Source: CAD feature listing. Evaluate the final solid. Frame: model axes, mm. A direction names the side the tool comes from. Round coordinates to 2 decimals unless told otherwise and drop trailing zeros. Order: outer loops, then holes, each group sorted by start corner. A loop starts at its lowest first (then second) coordinate and runs counter-clockwise, first axis right, second up. Notation, with made-up numbers: (-30, 19) -> (-4, 19) arc R20 cw to (-4, 39) -> close; hole circle Ø10 at (30.5, -7.75). An arc over 180 degrees is marked (long way). Answer as CSV lines item,"result".
from build123d import *

# Parameters (mm, degrees)
SKETCH1_W           = 17
SKETCH1_H           = 15
BOSS_EXTRUDE1_DEPTH = 81
CUT_EXTRUDE1_DEPTH  = 40
SKETCH3_R           = 1.5
CUT_EXTRUDE2_DEPTH  = 36
SKETCH4_W           = 17
SKETCH4_H           = 7
BOSS_EXTRUDE2_DEPTH = 14
SKETCH5_R           = 2
CUT_EXTRUDE3_DEPTH  = 14


with BuildPart() as part:
    # Sketch1 → Boss-Extrude1 (new body)
    with BuildSketch(Plane(origin=(0, 0, 0), x_dir=(1, 0, 0), z_dir=(0, 1, 0))):
        with Locations((-68.404761905, 8.571428571)):
            Rectangle(SKETCH1_W, SKETCH1_H)
    extrude(amount=BOSS_EXTRUDE1_DEPTH)

    # Sketch2 → Cut-Extrude1 (cut)
    with BuildSketch(Plane(origin=(-59.904761905, 0, 0), x_dir=(0, 0, -1), z_dir=(1, 0, 0))):
        Polygon((16.071428571, 0), (1.071428571, 0), (1.071428571, 6.994614872), align=None)
    extrude(amount=-CUT_EXTRUDE1_DEPTH, mode=Mode.SUBTRACT)

    # Sketch3 → Cut-Extrude2 (cut)
    with BuildSketch(Plane(origin=(0, 6.155714275, -2.870456708), x_dir=(1, 0, 0), z_dir=(0, -0.9063077870366528, 0.4226182617406934))):
        with Locations(Location((-68.404761905, -5.514992079, 0), (0, 0, 270))):
            Circle(SKETCH3_R)
    extrude(amount=-CUT_EXTRUDE2_DEPTH, mode=Mode.SUBTRACT)

    # Sketch4 → Boss-Extrude2 (add)
    with BuildSketch(Plane(origin=(0, 0, -16.071428571), x_dir=(-1, 0, 0), z_dir=(0, 0, -1))):
        with Locations((68.404761905, 77.5)):
            Rectangle(SKETCH4_W, SKETCH4_H)
    extrude(amount=BOSS_EXTRUDE2_DEPTH)

    # Sketch5 → Cut-Extrude3 (cut)
    with BuildSketch(Plane(origin=(0, 74, 0), x_dir=(-1, 0, 0), z_dir=(0, -1, 0))):
        with Locations(Location((71.904761905, 23.071428571, 0), (0, 0, 90))):
            Circle(SKETCH5_R)
        with Locations(Location((64.904761905, 23.071428571, 0), (0, 0, 90))):
            Circle(SKETCH5_R)
    extrude(amount=-CUT_EXTRUDE3_DEPTH, mode=Mode.SUBTRACT)


solid = part.part
1. Mould query, pull axis X, two halves, no side actions, for faces 1 (the flat face through (-59.905, 49, -9)), 2 (the flat face through (-76.905, 49, -9)), 3 (the cylindrical face through (-68.339, 12.335, -10.184)), 4 (the cylindrical face through (-66.857, 77.451, -22.638)). Classes: released by +X, released by -X, zero draft, split by the parting line, or undercut.
Results below:
face 1,"released by +X"
face 2,"released by -X"
face 3,"undercut"
face 4,"undercut"
2. Section query C-C on y = 59. Return loops of the section in (x, z).
Results below:
outline,"(-76.9, -16.07) -> (-59.9, -16.07) -> (-59.9, -1.07) -> (-76.9, -1.07) -> close"
3. Reachability of faces 5 (the cylindrical face through (-73.857, 77.451, -22.638)), 6 (the flat face through (-68, 74, -23)) from +Z, -Z, +X, -X, +Y, -Y: full face, straight path, thin tool, end or side. Return the list, or none.
Results below:
face 5,"+Y, -Y"
face 6,"-Z, +X, -X, -Y"
4. Line query: L1, parallel to Y at x = -68, z = -22.75; L2, parallel to Z at x = -63.5, y = 31.5; L3, parallel to Z at x = -67.25, y = 4.5. Output: solid intervals per line, ascending. Write a range as [from, to].
Results below:
L1,"[74, 81]"
L2,"[-16.07, -1.07]"
L3,"[-16.07, -9.24], [-7.13, -6.42]"
5. Section query A-A on z = -23.5. Return loops of the section in (x, y), and give its area (3 significant figures).
Results below:
outline,"(-76.9, 74) -> (-73.86, 74) -> (-73.86, 81) -> (-76.9, 81) -> close; (-69.95, 74) -> (-66.86, 74) -> (-66.86, 81) -> (-69.95, 81) -> close; (-62.95, 74) -> (-59.9, 74) -> (-59.9, 81) -> (-62.95, 81) -> close"
area,"64.3 mm2"
6. Section query D-D on z = -27.75. Return loops of the section in (x, y), and give its area (3 significant figures).
Results below:
outline,"(-76.9, 74) -> (-59.9, 74) -> (-59.9, 81) -> (-76.9, 81) -> close"
area,"119 mm2"
7. Pin query (flat end, axial travel): pin 1 (2 mm diameter, centred on x = -68.5, y = 28, fed in from -Z); pin 2 (3 mm diameter, centred on x = -64.9, z = -23.07, fed in from -Y); pin 3 (5 mm diameter, centred on x = -70.5, z = -23.5, fed in from -Y). Return the tip coordinate at first contact, or that it passes through.
Results below:
pin 1,"z = -16.07"
pin 2,"through"
pin 3,"y = 74"
8. Section query B-B on x = -76. Return loops of the section in (y, z), and give its area (3 significant figures).
Results below:
outline,"(0, -16.07) -> (74, -16.07) -> (74, -30.07) -> (81, -30.07) -> (81, -1.07) -> (6.99, -1.07) -> close"
area,"1,260 mm2"
